Geometry check sheet. Reference: the model listing, model coordinates, mm. A direction names the side the tool comes from. Round coordinates to 2 decimals unless told otherwise and drop trailing zeros. Write each loop counter-clockwise with the first axis right and the second up, starting at its lowest first coordinate (ties: lowest second). Pieces come first, ordered by that corner, then holes. Notation, with made-up numbers: M 38.5,-2 L 44.5,-2 A16 ccw 44.5,8 Z; hole C 52.5,-8 d9. An arc over 180 degrees is marked long. Use a Markdown table: item, result.
```python
from build123d import *

# Parameters (mm, degrees)
F0_R      = 6.6675
F1_DEPTH  = 4.7625
F2_W      = 6.35
F2_H      = 66.675
F3_DEPTH  = 63.5
F4_R      = 7.9375
F4_W      = 63.5
F4_H      = 25.4
F5_DEPTH  = 87.4548256
F7_DEPTH  = 4.7625
F8_W      = 28.575
F8_H      = 4.7625
F9_REACH  = 92.4701565505
F11_REACH = 103.9121525448
F13_DEPTH = 98.6684645933


with BuildPart() as f1:
    # F0 (on Front) → F1 (new body)
    with BuildSketch(Plane.XZ):
        Polygon((-67.6469967966, 97.79), (-146.05, 82.55), (-146.05, -13.5774645933), (-69.85, -13.5774645933), (0, 0), (0, 97.79), align=None)
        with Locations((-127, 8.89)):
            Circle(F0_R, mode=Mode.SUBTRACT)
        with Locations((-19.05, 8.89)):
            Circle(F0_R, mode=Mode.SUBTRACT)
        with Locations((-127, 72.39)):
            Circle(F0_R, mode=Mode.SUBTRACT)
        with Locations((-63.5, 72.39)):
            Circle(F0_R, mode=Mode.SUBTRACT)
    extrude(amount=F1_DEPTH)

    # F2 (on face) → F3 (join)
    with BuildSketch(Plane(origin=(0, 0, 0), x_dir=(-1, 0, 0), z_dir=(0, 1, 0))):
        with Locations((45.5438256, 58.7375)):
            Rectangle(F2_W, F2_H)
        with Locations((84.2788256, 58.7375)):
            Rectangle(F2_W, F2_H)
    extrude(amount=F3_DEPTH)

    # F4 (on face) → F5 (cut, through all)
    with BuildSketch(Plane(origin=(-87.4538256, 0, 0), x_dir=(0, -1, 0), z_dir=(-1, 0, 0))):
        Polygon((-63.5, 79.375), (0, 92.075), (-63.5, 92.075), align=None)
        with Locations((-50.8, 66.675)):
            Circle(F4_R)
        with Locations((-31.75, 38.1)):
            Rectangle(F4_W, F4_H)
    extrude(amount=-F5_DEPTH, mode=Mode.SUBTRACT)

    # F6 (on face) → F7 (join)
    with BuildSketch(Plane(origin=(0, 17.7067307692, 88.5336538462), x_dir=(1, 0, 0), z_dir=(0, 0.1961161351, 0.9805806757))):
        with BuildLine():
            Line((-87.4538256, -13.2948931428), (-42.3688256, -13.2948931428))
            Line((-42.3688256, -13.2948931428), (-42.3688256, 21.6301068572))
            Line((-42.3688256, 21.6301068572), (-53.4813256, 21.6301068572))
            ThreePointArc((-53.4813256, 21.6301068572), (-64.9113256, 18.9130321535), (-76.3413256, 21.6301068572))
            Line((-76.3413256, 21.6301068572), (-87.4538256, 21.6301068572))
            Line((-87.4538256, 21.6301068572), (-87.4538256, -13.2948931428))
        make_face()
    extrude(amount=F7_DEPTH)

    f9_end = Plane(origin=(-47.9250756, 39.3837971133, 86.6266486207), x_dir=(0, 0.1961161351, 0.9805806757), z_dir=(0, 0.9805806757, -0.1961161351))
    # F8 (on face) → F9 (join, up to a plane its end follows)
    with BuildSketch(Plane(origin=(0, 0, 0), x_dir=(-1, 0, 0), z_dir=(0, 1, 0))):
        with Locations((28.0813256, 82.70875)):
            Rectangle(F8_W, F8_H)
        with Locations((101.7413256, 82.70875)):
            Rectangle(F8_W, F8_H)
    f9_long = extrude(amount=F9_REACH, mode=Mode.PRIVATE)
    add(split(f9_long, bisect_by=f9_end, keep=Keep.BOTTOM, mode=Mode.PRIVATE))

    f11_end = Plane(origin=(-33.5594638675, 38.8165352763, 83.7903394356), x_dir=(0, 0.1961161351, 0.9805806757), z_dir=(0, 0.9805806757, -0.1961161351))
    # F10 (on face) → F11 (join, up to a plane its end follows)
    with BuildSketch(Plane(origin=(0, 0, 0), x_dir=(-1, 0, 0), z_dir=(0, 1, 0))):
        Polygon((20.5290176908, 80.3275), (13.7938256, 80.3275), (42.3688256, 51.7525), (42.3688256, 58.4876920908), align=None)
        Polygon((116.0288256, 80.3275), (109.2936335092, 80.3275), (87.4538256, 58.4876920908), (87.4538256, 51.7525), align=None)
    f11_long = extrude(amount=F11_REACH, mode=Mode.PRIVATE)
    add(split(f11_long, bisect_by=f11_end, keep=Keep.BOTTOM, mode=Mode.PRIVATE))

    # F12 (on face) → F13 (cut, through all)
    with BuildSketch(Plane.XY.offset(85.09)):
        Polygon((-13.7938256, 39.0764673892), (-32.8438256, 39.0764673892), (-13.7938256, 20.0264673892), align=None)
        Polygon((-116.0288256, 20.0264673892), (-96.9788256, 39.0764673892), (-116.0288256, 39.0764673892), align=None)
    extrude(amount=-F13_DEPTH, mode=Mode.SUBTRACT)


solid = f1.part
```
Item 1: Material ranges on line 1 along Z through (x, y) = (-63.5, -2.55); line 2 along Z through (x, y) = (-35.5, 18.5); line 3 along Y through (x, z) = (-41, 92.5), recorded low to high. Write a range as from..to.
Outcome:
| item | result |
|---|---|
| line 1 | z = -12.34..65.72, 79.06..97.79 |
| line 2 | z = 58.62..65.36, 80.33..85.09 |
| line 3 | y = -4.76..0 |
Item 2: Cross-section at C-C, the plane x = -127. Record the cut outline in (y, z).
Outcome:
| item | result |
|---|---|
| outline | M -4.76,-13.58 L 0,-13.58 L 0,2.22 L -4.76,2.22 Z; M -4.76,15.56 L 0,15.56 L 0,65.72 L -4.76,65.72 Z; M -4.76,79.06 L 0,79.06 L 0,86.25 L -4.76,86.25 Z |
Item 3: Go/stop test with flat-tipped pins: pin 1 (5 mm diameter, centred on y = 6, z = 83, fed in from +X); pin 2 (4 mm diameter, centred on x = -40.5, y = 41.5, fed in from -Z); pin 3 (10 mm diameter, centred on y = 45.5, z = 75, fed in from -X); pin 4 (9.5 mm diameter, centred on y = 50.8, z = 66.675, fed in from +X). Record where each tip stops, or that it passes through.
Outcome:
| item | result |
|---|---|
| pin 1 | stops at x = -13.79 |
| pin 2 | stops at z = 50.8 |
| pin 3 | stops at x = -87.45 |
| pin 4 | passes through |
Item 4: Access from +Z, -Z, +X, -X, +Y, -Y to the whole of each face (thin tool, end or side, straight path). Record for faces 4 (the face through (-98.527, 17.862, 69.56)), 5 (the face through (-65.23, 5.13, 93.44)), 6 (the face through (-35.59, 34.31, 61.26)), 7 (the face through (-13.794, 10, 83)).
Outcome:
| item | result |
|---|---|
| face 4 | +Y |
| face 5 | +Z, +X, -X |
| face 6 | -Z, +X, +Y |
| face 7 | +Z, -Z, +X, +Y |
Item 5: Cross-section at B-B, the plane y = 50.8. Record the cut outline in (x, z) (1 decimal).
Outcome:
| item | result |
|---|---|
| outline | M -87.5,50.8 L -81.1,50.8 L -81.1,58.7 L -87.5,58.7 Z; M -87.5,74.6 L -81.1,74.6 L -81.1,81.9 L -87.5,81.9 Z; M -48.7,50.8 L -42.4,50.8 L -42.4,58.7 L -48.7,58.7 Z; M -48.7,74.6 L -42.4,74.6 L -42.4,81.9 L -48.7,81.9 Z |
Item 6: Cross-section at D-D, the plane y = 10. Record the cut outline in (x, z) (1 decimal), and give its area (3 significant figures).
Outcome:
| item | result |
|---|---|
| outline | M -116,80.3 L -87.5,51.8 L -87.5,50.8 L -81.1,50.8 L -81.1,90.1 L -48.7,90.1 L -48.7,50.8 L -42.4,50.8 L -42.4,51.8 L -13.8,80.3 L -13.8,85.1 L -42.4,85.1 L -42.4,94.9 L -87.5,94.9 L -87.5,85.1 L -116,85.1 Z; hole M -109.3,80.3 L -87.5,58.5 L -87.5,80.3 Z; hole M -42.4,58.5 L -20.5,80.3 L -42.4,80.3 Z |
| area | 1,330 mm2 |
Item 7: Mould release check, pull along X, two halves, no side actions. Record for faces 1 (the face through (-34, 0, 72)), 2 (the face through (-65.227, 22.967, 92.338)), 3 (the face through (-42.369, 15, 89)): +X half, -X half, draft (parallel to the pull), parting line (faces both ways), or undercut.
Outcome:
| item | result |
|---|---|
| face 1 | undercut |
| face 2 | draft |
| face 3 | +X half |
Item 8: Cross-section at A-A, the plane z = 8.89. Record the cut outline in (x, y).
Outcome:
| item | result |
|---|---|
| outline | M -146.05,-4.76 L -133.67,-4.76 L -133.67,0 L -146.05,0 Z; M -120.33,-4.76 L -25.72,-4.76 L -25.72,0 L -120.33,0 Z; M -12.38,-4.76 L 0,-4.76 L 0,0 L -12.38,0 Z |
